For this review, take the finished solid that the model builds, in its own axes (mm). Face numbers are marked on the shaded views. Give positions to 0.01 mm unless a question says otherwise; leave off trailing zeros. Write each loop counter-clockwise with the first axis right and the second up, starting at its lowest first coordinate (ties: lowest second). Pieces come first, ordered by that corner, then holes. Notation, with made-up numbers: M 63.5,13.5 L 121.5,13.5 A16 ccw 121.5,33.5 Z; hole C 58,61.25 d1. An arc over 180 degrees is marked long. Write item = value, one per line.
```python
from build123d import *

# Parameters (mm, degrees)
SKETCH1_W                                  = 55
SKETCH1_H                                  = 500
BOSS_EXTRUDE1_DEPTH                        = 110
SKETCH2_W                                  = 15
SKETCH2_H                                  = 45
CUT_EXTRUDE1_DEPTH                         = 500
M10X1_0_TAPPED_HOLE1_D                     = 9
M10X1_0_TAPPED_HOLE1_DEPTH                 = 23
M10X1_0_TAPPED_HOLE1_CBORE_D               = 10
M10X1_0_TAPPED_HOLE1_CBORE_DEPTH           = 20
M10X1_0_TAPPED_HOLE1_TIP                   = 2.703872786
M10X1_0_TAPPED_HOLE2_D                     = 9
M10X1_0_TAPPED_HOLE2_DEPTH                 = 23
M10X1_0_TAPPED_HOLE2_CBORE_D               = 10
M10X1_0_TAPPED_HOLE2_CBORE_DEPTH           = 20
M10X1_0_TAPPED_HOLE2_TIP                   = 2.703872786
M10X1_0_TAPPED_HOLE2_ON_FACE_2_D           = 9
M10X1_0_TAPPED_HOLE2_ON_FACE_2_DEPTH       = 23
M10X1_0_TAPPED_HOLE2_ON_FACE_2_CBORE_D     = 10
M10X1_0_TAPPED_HOLE2_ON_FACE_2_CBORE_DEPTH = 20
M10X1_0_TAPPED_HOLE2_ON_FACE_2_TIP         = 2.703872786


with BuildPart() as part:
    # Sketch1 → Boss-Extrude1 (new body)
    with BuildSketch(Plane(origin=(0, 0, 0), x_dir=(1, 0, 0), z_dir=(0, 1, 0))):
        with Locations((24.098703387, 215.534456811)):
            Rectangle(SKETCH1_W, SKETCH1_H)
    extrude(amount=BOSS_EXTRUDE1_DEPTH)

    # Sketch2 → Cut-Extrude1 (cut)
    with BuildSketch(Plane.XY.offset(34.465543189)):
        with Locations((16.598703387, 77.5)):
            Rectangle(SKETCH2_W, SKETCH2_H)
        with Locations((31.598703387, 77.5)):
            Rectangle(SKETCH2_W, SKETCH2_H)
        with Locations((31.598703387, 32.5)):
            Rectangle(SKETCH2_W, SKETCH2_H)
        with Locations((16.598703387, 32.5)):
            Rectangle(SKETCH2_W, SKETCH2_H)
    extrude(amount=-CUT_EXTRUDE1_DEPTH, mode=Mode.SUBTRACT)

    # M10x1.0 Tapped Hole1
    with Locations(Plane(origin=(0, 10, 0), x_dir=(1, 0, 0), z_dir=(0, 1, 0))):
        with Locations((24.098703387, 450.534456811), (24.098703387, -19.465543189)):
            CounterBoreHole(M10X1_0_TAPPED_HOLE1_D / 2, M10X1_0_TAPPED_HOLE1_CBORE_D / 2, M10X1_0_TAPPED_HOLE1_CBORE_DEPTH, depth=M10X1_0_TAPPED_HOLE1_DEPTH)
            with Locations((0, 0, -(M10X1_0_TAPPED_HOLE1_DEPTH + M10X1_0_TAPPED_HOLE1_TIP / 2))):  # 118° drill point
                Cone(0, M10X1_0_TAPPED_HOLE1_D / 2, M10X1_0_TAPPED_HOLE1_TIP, mode=Mode.SUBTRACT)

    # M10x1.0 Tapped Hole2
    with Locations(Plane(origin=(51.598703387, 85, -450.534456811), x_dir=(0, 0, 1), z_dir=(1, 0, 0))):
        with Locations((0, 0), (0, 60), (470, 0), (470, 60)):
            CounterBoreHole(M10X1_0_TAPPED_HOLE2_D / 2, M10X1_0_TAPPED_HOLE2_CBORE_D / 2, M10X1_0_TAPPED_HOLE2_CBORE_DEPTH, depth=M10X1_0_TAPPED_HOLE2_DEPTH)
            with Locations((0, 0, -(M10X1_0_TAPPED_HOLE2_DEPTH + M10X1_0_TAPPED_HOLE2_TIP / 2))):  # 118° drill point
                Cone(0, M10X1_0_TAPPED_HOLE2_D / 2, M10X1_0_TAPPED_HOLE2_TIP, mode=Mode.SUBTRACT)

    # M10x1.0 Tapped Hole2 on face 2
    with Locations(Plane(origin=(233.947763792, 74.109982143, 0), x_dir=(0, 0, 1), z_dir=(1, 0, 0))):
        with Locations((0, 0)):
            CounterBoreHole(M10X1_0_TAPPED_HOLE2_ON_FACE_2_D / 2, M10X1_0_TAPPED_HOLE2_ON_FACE_2_CBORE_D / 2, M10X1_0_TAPPED_HOLE2_ON_FACE_2_CBORE_DEPTH, depth=M10X1_0_TAPPED_HOLE2_ON_FACE_2_DEPTH)
            with Locations((0, 0, -(M10X1_0_TAPPED_HOLE2_ON_FACE_2_DEPTH + M10X1_0_TAPPED_HOLE2_ON_FACE_2_TIP / 2))):  # 118° drill point
                Cone(0, M10X1_0_TAPPED_HOLE2_ON_FACE_2_D / 2, M10X1_0_TAPPED_HOLE2_ON_FACE_2_TIP, mode=Mode.SUBTRACT)


solid = part.part
```
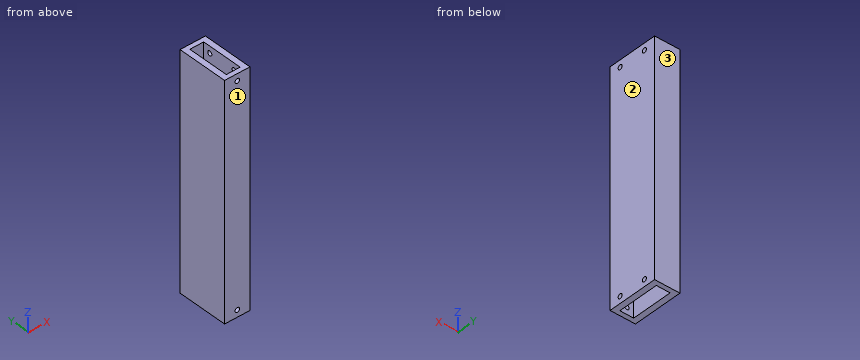
1. For line 1 along Z through (x, y) = (43.25, 25); line 2 along Y through (x, z) = (35, -118); line 3 along X through (y, z) = (51, -227.5), list the stretches that pass through material, from the lowest coordinate up. Write a range as from..to.
Responses:
line_1 = -465.53..-455.53, -445.53..14.47, 24.47..34.47
line_2 = 0..10, 100..110
line_3 = -3.4..9.1, 39.1..51.6
2. The part is to be moulded in two halves that separate along Y. For the marked faces 1, 2 and 3, say which applies: +Y half, -Y half, draft (parallel to the pull), parting line (faces both ways), or undercut.
Responses:
face_1 = -Y half
face_2 = draft
face_3 = +Y half
3. We need section B-B, the plane z = -135. Write out the cut boundary in (x, y), then the cut area to 3 significant figures.
Responses:
outline = M -3.4,0 L 51.6,0 L 51.6,110 L -3.4,110 Z; hole M 9.1,10 L 39.1,10 L 39.1,100 L 9.1,100 Z
area = 3,350 mm2
4. Insertion check: P1, Ø9, axis at x = 24.1, z = 19.47, coming from the -Y side; P2, Ø9, axis at y = 25, z = 19.47, coming from the +X side; P3, Ø5, axis at x = 35.5, y = 80, coming from the -Z side. Each pin has a flat end and moves straight along its axis. Give the tip position at first contact, or say it passes through.
Responses:
P1 = 100
P2 = 9.1
P3 = through
5. We need section A-A, the plane y = 58. Write out the cut boundary in (x, z), then the cut area to 3 significant figures.
Responses:
outline = M -3.4,-465.53 L 9.1,-465.53 L 9.1,34.47 L -3.4,34.47 Z; M 39.1,-465.53 L 51.6,-465.53 L 51.6,34.47 L 39.1,34.47 Z
area = 12,500 mm2
6. We need section C-C, the plane y = 85. Write out the cut boundary in (x, z).
Responses:
outline = M -3.4,-465.53 L 9.1,-465.53 L 9.1,34.47 L -3.4,34.47 Z; M 39.1,-465.53 L 51.6,-465.53 L 51.6,-455.53 L 39.1,-455.53 Z; M 39.1,-445.53 L 51.6,-445.53 L 51.6,14.47 L 39.1,14.47 Z; M 39.1,24.47 L 51.6,24.47 L 51.6,34.47 L 39.1,34.47 Z
